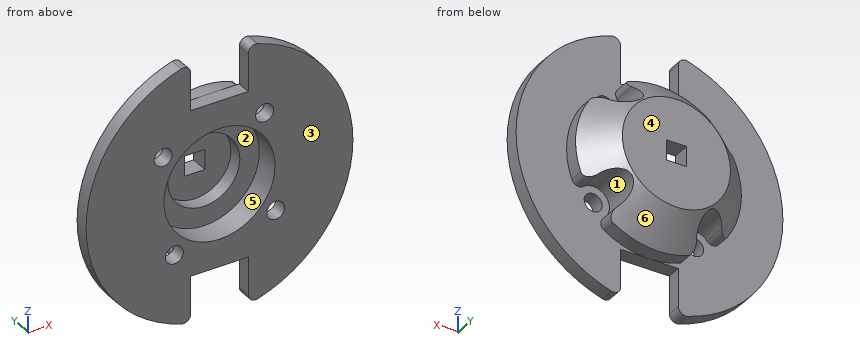
```python
from build123d import *

# Parameters (mm, degrees)
SKETCH1_R             = 12.5
BOSS_EXTRUDE1_DEPTH   = 2
SKETCH2_R             = 11.5
BOSS_EXTRUDE2_DEPTH   = 6
F_2_5MM_DOWEL_HOLE1_D = 2.5
SKETCH7_R             = 2.25
CUT_EXTRUDE1_DEPTH    = 15
CIRPATTERN1_COUNT     = 4
SKETCH8_R             = 7.7
CUT_EXTRUDE2_DEPTH    = 3.5
CHAMFER4_SIZE         = 4
SKETCH3_W             = 2.8
SKETCH3_H             = 2.8
CUT_EXTRUDE3_DEPTH    = 20.403607912
SKETCH9_R             = 5
CUT_EXTRUDE4_DEPTH    = 2
FILLET1_R             = 1
SKETCH11_W            = 6
SKETCH11_H            = 2
SKETCH13_W            = 8
SKETCH13_H            = 10.327587527
CUT_EXTRUDE5_DEPTH    = 10
FILLET2_R             = 1


with BuildPart() as part:
    # Sketch1 → Boss-Extrude1 (new body)
    with BuildSketch(Plane(origin=(0, 0, 0), x_dir=(1, 0, 0), z_dir=(0, 1, 0))):
        with Locations(Location((0, 0, 0), (0, 0, 270))):
            Circle(SKETCH1_R)
    extrude(amount=BOSS_EXTRUDE1_DEPTH)

    # Sketch2 → Boss-Extrude2 (add)
    with BuildSketch(Plane(origin=(0, 2, 0), x_dir=(1, 0, 0), z_dir=(0, 1, 0))):
        with Locations(Location((0, 0, 0), (0, 0, 270))):
            Circle(SKETCH2_R)
    extrude(amount=BOSS_EXTRUDE2_DEPTH)

    # Ø2.5mm Dowel Hole1 (through all)
    with Locations(Plane(origin=(0, 0, 0), x_dir=(-1, 0, 0), z_dir=(0, -1, 0))):
        with Locations((-6.252229289, -7.804462116)):
            f_2_5mm_dowel_hole1 = Hole(F_2_5MM_DOWEL_HOLE1_D / 2)

    # Sketch7 → Cut-Extrude1 (cut)
    with BuildSketch(Plane(origin=(0, 2, 0), x_dir=(1, 0, 0), z_dir=(0, 1, 0))):
        with Locations((6.252229289, -7.804462116)):
            Circle(SKETCH7_R)
    cut_extrude1 = extrude(amount=CUT_EXTRUDE1_DEPTH, mode=Mode.SUBTRACT)

    # CirPattern1: Ø2.5mm Dowel Hole1, Cut-Extrude1 ×4 about axis
    cirpattern1_axis = Axis((0, 0, 0), (0, 1, 0))
    add([f_2_5mm_dowel_hole1.rotate(cirpattern1_axis, i * 360 / CIRPATTERN1_COUNT) for i in range(1, CIRPATTERN1_COUNT)], mode=Mode.SUBTRACT)
    add([cut_extrude1.rotate(cirpattern1_axis, i * 360 / CIRPATTERN1_COUNT) for i in range(1, CIRPATTERN1_COUNT)], mode=Mode.SUBTRACT)

    # Sketch8 → Cut-Extrude2 (cut)
    with BuildSketch(Plane.XZ):
        with Locations(Location((0, 0, 0), (0, 0, 270))):
            Circle(SKETCH8_R)
    extrude(amount=-CUT_EXTRUDE2_DEPTH, mode=Mode.SUBTRACT)

    # Chamfer4
    # the kernel refuses this chamfer: 4 mm, written as the material it takes off along each edge
    with BuildSketch(Plane(origin=(0, 8, 0), x_dir=(-0.15654942512802536, 0, 0.9876701258477371), z_dir=(0.9876701258477371, 0, 0.15654942512802536))) as chamfer4_piece_1:
        Polygon((11.5, CHAMFER4_SIZE), (11.5 - CHAMFER4_SIZE, 0), (11.5, 0), align=None)
    revolve(axis=Axis((0, 8, 0), (0, -1, 0)), revolution_arc=174.589558781, mode=Mode.SUBTRACT)
    with BuildSketch(Plane(origin=(0, 8, 0), x_dir=(0.9876701258477374, 0, 0.15654942512802353), z_dir=(0.15654942512802353, 0, -0.9876701258477374))) as chamfer4_piece_2:
        Polygon((11.5, CHAMFER4_SIZE), (11.5 - CHAMFER4_SIZE, 0), (11.5, 0), align=None)
    revolve(axis=Axis((0, 8, 0), (0, -1, 0)), revolution_arc=174.589558781, mode=Mode.SUBTRACT)
    with BuildSketch(Plane(origin=(0, 8, 0), x_dir=(-0.9876701258477374, 0, -0.15654942512802342), z_dir=(-0.15654942512802342, 0, 0.9876701258477374))) as chamfer4_piece_3:
        Polygon((11.5, CHAMFER4_SIZE), (11.5 - CHAMFER4_SIZE, 0), (11.5, 0), align=None)
    revolve(axis=Axis((0, 8, 0), (0, -1, 0)), revolution_arc=174.589558781, mode=Mode.SUBTRACT)
    with BuildSketch(Plane(origin=(0, 8, 0), x_dir=(0.15654942512802555, 0, -0.987670125847737), z_dir=(-0.987670125847737, 0, -0.15654942512802555))) as chamfer4_piece_4:
        Polygon((11.5, CHAMFER4_SIZE), (11.5 - CHAMFER4_SIZE, 0), (11.5, 0), align=None)
    revolve(axis=Axis((0, 8, 0), (0, -1, 0)), revolution_arc=174.589558781, mode=Mode.SUBTRACT)

    # Sketch3 → Cut-Extrude3 (cut, through all)
    with BuildSketch(Plane(origin=(0, 8, 0), x_dir=(1, 0, 0), z_dir=(0, 1, 0))):
        Rectangle(SKETCH3_W, SKETCH3_H)
    extrude(amount=-CUT_EXTRUDE3_DEPTH, mode=Mode.SUBTRACT)

    # Sketch9 → Cut-Extrude4 (cut)
    with BuildSketch(Plane.XZ.offset(-3.5)):
        with Locations(Location((0, 0, 0), (0, 0, 270))):
            Circle(SKETCH9_R)
    extrude(amount=-CUT_EXTRUDE4_DEPTH, mode=Mode.SUBTRACT)

    # Fillet1
    # the kernel refuses this fillet: 1 mm, written as the material it takes off along each edge
    with BuildSketch(Plane(origin=(-7.744399955, 8.541870217, 8.501427488), x_dir=(0.7901380360957252, 0, 0.6129289387154032), z_dir=(0, -1, 0)), Plane(origin=(-8.501427488, 8.541870217, -7.744399955), x_dir=(-0.6129289387154034, 0, 0.790138036095725), z_dir=(0, -1, 0)), Plane(origin=(8.501427488, 8.541870217, 7.744399955), x_dir=(0.6129289387154006, 0, -0.7901380360957272), z_dir=(0, -1, 0))) as fillet1_piece_1:
        with BuildLine():
            CenterArc((1.73775904, -0.996875484), FILLET1_R, 85.469541484, 107.754858312)
            ThreePointArc((0.76427747, -1.225640938), (0.48316298, -0.549824406), (0, 0))
            ThreePointArc((0, 0), (0.908374043, 0.035931935), (1.816748087, 0))
        make_face()
    extrude(amount=6.541870217, mode=Mode.SUBTRACT)
    with BuildSketch(Plane(origin=(-9.986362414, 8.541870217, 5.702855929), x_dir=(0.5425108766100752, 0, -0.840048777607448), z_dir=(0, -1, 0)), Plane(origin=(-5.702855929, 8.541870217, -9.986362414), x_dir=(0.8400487776074425, 0, 0.5425108766100841), z_dir=(0, -1, 0)), Plane(origin=(9.986362414, 8.541870217, -5.702855929), x_dir=(-0.5425108766100888, 0, 0.8400487776074392), z_dir=(0, -1, 0)), Plane(origin=(5.702855929, 8.541870217, 9.986362414), x_dir=(-0.8400487776074446, 0, -0.5425108766100806), z_dir=(0, -1, 0))) as fillet1_piece_2:
        with BuildLine():
            CenterArc((1.765388102, -0.94708609), FILLET1_R, 108.722180598, 107.754858312)
            ThreePointArc((0.961292932, -1.541586686), (0.450156717, -0.789805949), (0, 0))
            ThreePointArc((0, 0), (0.722204223, -0.119056298), (1.444408447, 0))
        make_face()
    extrude(amount=6.541870217, mode=Mode.SUBTRACT)
    with BuildSketch(Plane(origin=(7.744399955, 8.541870217, -8.501427488), x_dir=(-0.9381802645731545, 0, 0.34614706580505045), z_dir=(0, -1, 0))) as fillet1_piece_3:
        with BuildLine():
            CenterArc((1.765388102, 0.94708609), FILLET1_R, 143.52296109, 107.754858312)
            ThreePointArc((0.961292932, 1.541586686), (0.450156717, 0.789805949), (0, 0))
            ThreePointArc((0, 0), (0.722204223, 0.119056298), (1.444408447, 0))
        make_face()
    extrude(amount=6.541870217, mode=Mode.SUBTRACT)

    # Sketch11 → Revolve1 (revolve)
    with BuildSketch(Plane(origin=(0, 0, 0), x_dir=(0, 0, -1), z_dir=(1, 0, 0)), mode=Mode.PRIVATE) as revolve1_sk:
        with Locations((15.5, 1)):
            Rectangle(SKETCH11_W, SKETCH11_H)
    revolve(revolve1_sk.sketch.rotate(Axis((0, 0, 0), (0, 1, 0)), 20.668231864), axis=Axis((0, 0, 0), (0, 1, 0)))

    # Sketch13 → Cut-Extrude5 (cut)
    with BuildSketch(Plane(origin=(0, 2, 0), x_dir=(1, 0, 0), z_dir=(0, 1, 0))):
        with Locations((0, 16.663793764)):
            Rectangle(SKETCH13_W, SKETCH13_H)
        with Locations((0, -16.663793764)):
            Rectangle(SKETCH13_W, SKETCH13_H)
    extrude(amount=-CUT_EXTRUDE5_DEPTH, mode=Mode.SUBTRACT)

    # Fillet2
    fillet2_edges = [part.edges().sort_by_distance(p)[0] for p in [
        (-4, 1, -18.062391868),
        (4, 1, -18.062391868),
        (4, 1, 18.062391868),
        (-4, 1, 18.062391868),
    ]]
    fillet(fillet2_edges, radius=FILLET2_R)


solid = part.part
```
CAD build for the part. Positions are in the model's coordinates, mm. Face numbers are marked on the shaded views. A direction names the side the tool comes from. Coordinates: 2 decimals unless noted, no trailing zeros. Write each loop counter-clockwise with the first axis right and the second up, starting at its lowest first coordinate (ties: lowest second). Pieces come first, ordered by that corner, then holes. Notation, with made-up numbers: (-17.5, -36) -> (25.5, -36) arc R14 ccw to (25.5, -11) -> close; hole circle Ø5 at (-36.5, -25). An arc over 180 degrees is marked (long way). Return JSON: item names as keys, results as strings. Group by question number.
Q1. Pull direction Z, two halves, no side cores. Call the marked faces 4, 5 and 6: released by +Z, released by -Z, zero draft, split by the parting line, or undercut.
Q2. Cut at D-D, the plane y = 6.75. Give the cut face in (x, z), then the cut area to 3 significant figures.
Q3. Which spindle directions (+Z, -Z, +X, -X, +Y, -Y) get a long thin tool onto all of the face, cutting with end or side? Do the marked faces 1, 2 and 3. Say none if no direction does.
Q4. Cut at B-B, the plane y = 2.5. Give the cut face in (x, z), then the cut area to 3 significant figures.
Q5. Cut at C-C, the plane x = -12. Give the cut face in (y, z), then the cut area to 3 significant figures.
Q6. Drill centre lines: line 1 (Y direction, x = -9, z = -11.5); line 2 (Z direction, x = 3.5, y = 5); line 3 (X direction, y = 2.15, z = 0). Where is each one in solid material? Low to high.
Q7. Flat gauge pins, fed straight in: pin 1 (2 mm diameter, centred on y = 6.5, z = -0.5, fed in from -X); pin 2 (1 mm diameter, centred on x = -2, y = 1, fed in from +Z); pin 3 (2 mm diameter, centred on x = 0.5, y = 6.5, fed in from -Z). Where does each tip first touch, or does it go through?
Q8. Cut at A-A, the plane z = 0. Give the cut face in (x, y).
Returned:
{
 "1": {"face 4": "zero draft", "face 5": "undercut", "face 6": "split by the parting line"},
 "2": {"outline": "(-7.78, 4) arc R8.75 ccw to (-6.72, -5.6) arc R2.25 cw to (-4, -7.78) arc R8.75 ccw to (5.6, -6.72) arc R2.25 cw to (7.78, -4) arc R8.75 ccw to (6.72, 5.6) arc R2.25 cw to (4, 7.78) arc R8.75 ccw to (-5.6, 6.72) arc R2.25 cw to start; hole (-1.4, -1.4) -> (1.4, -1.4) -> (1.4, 1.4) -> (-1.4, 1.4) -> close", "area": "223 mm2"},
 "3": {"face 1": "+Y", "face 2": "-Y", "face 3": "+Z, -Z, +X, -X, -Y"},
 "4": {"outline": "(-10.76, 4.06) arc R11.5 ccw to (-9.61, -6.31) arc R1 ccw to (-8, -6.39) arc R2.25 cw to (-4.49, -9.2) arc R1 ccw to (-4.06, -10.76) arc R11.5 ccw to (6.31, -9.61) arc R1 ccw to (6.39, -8) arc R2.25 cw to (9.2, -4.49) arc R1 ccw to (10.76, -4.06) arc R11.5 ccw to (9.61, 6.31) arc R1 ccw to (8, 6.39) arc R2.25 cw to (4.49, 9.2) arc R1 ccw to (4.06, 10.76) arc R11.5 ccw to (-6.31, 9.61) arc R1 ccw to (-6.39, 8) arc R2.25 cw to (-9.2, 4.49) arc R1 ccw to start; hole circle Ø15.4 at (0, 0)", "area": "169 mm2"},
 "5": {"outline": "(0, -14.08) -> (2, -14.08) -> (2, 14.08) -> (0, 14.08) -> close", "area": "56.3 mm2"},
 "6": {"line 1": "y = 0 to 2", "line 2": "z = -9.9 to -3.57, 3.57 to 9.9", "line 3": "x = -11.5 to -7.7, 7.7 to 11.5"},
 "7": {"pin 1": "stops at x = -9.99", "pin 2": "stops at z = 11.5", "pin 3": "stops at z = -9.99"},
 "8": {"outline": "(-18.5, 0) -> (-7.7, 0) -> (-7.7, 3.5) -> (-5, 3.5) -> (-5, 5.5) -> (-1.4, 5.5) -> (-1.4, 8) -> (-7.5, 8) -> (-11.5, 4) -> (-11.5, 2) -> (-18.5, 2) -> close; (1.4, 5.5) -> (5, 5.5) -> (5, 3.5) -> (7.7, 3.5) -> (7.7, 0) -> (18.5, 0) -> (18.5, 2) -> (11.5, 2) -> (11.5, 4) -> (7.5, 8) -> (1.4, 8) -> close"}
}
